Source: three-view drawing plus pictorial views. Frame: mm from the lowest corner of the part. A direction names the side the tool comes from. Coordinates: 2 decimals unless noted, no trailing zeros. Order: outer loops, then holes, each group sorted by start corner. A loop starts at its lowest first (then second) coordinate and runs counter-clockwise, first axis right, second up. Notation, with made-up numbers: M 61,-6 L 91,-6 A24 ccw 91,23 Z; hole C 2.25,54.25 d4. An arc over 180 degrees is marked long. Use CSV: the item, a comma, the result in double quotes. Start each with the question number.
Q1. Section query C-C, the plane x = 10.5. Output: boundary loops of the cut face in (y, z).
Q2. First-contact query: P1, Ø16, axis at x = 26, z = 25, coming from the +Y side; P2, Ø3, axis at x = 18, z = 24.5, coming from the -Y side. Flat tips, straight axial feed; report the tip coordinate or a pass-through.
Q3. Ray query, probe 1 along Y at (x, z) = (30, 7.5); probe 2 along X at (y, z) = (25, 12); probe 3 along Y at (x, z) = (34, 25.5). Return the intervals inside material, ascending.
Q4. Section query B-B, the plane z = 25. Output: boundary loops of the cut face in (x, y).
Q5. Section query D-D, the plane y = 16.5. Output: boundary loops of the cut face in (x, z), and give its area (3 significant figures).
Q6. Access query for the marked faces 1, 2 and 3. Directions: +Z, -Z, +X, -X, +Y, -Y. A direction counts if a zero-diameter tool reaches every point of the face in a straight line with its end or side. Return the directions, or none.
Q7. Section query A-A, the plane x = 26. Output: boundary loops of the cut face in (y, z).
Q8. Mould query, pull axis Y, two halves, no side actions, for the marked faces 4, 5 and 6. Classes: +Y half, -Y half, draft (parallel to the pull), parting line (faces both ways), or undercut.
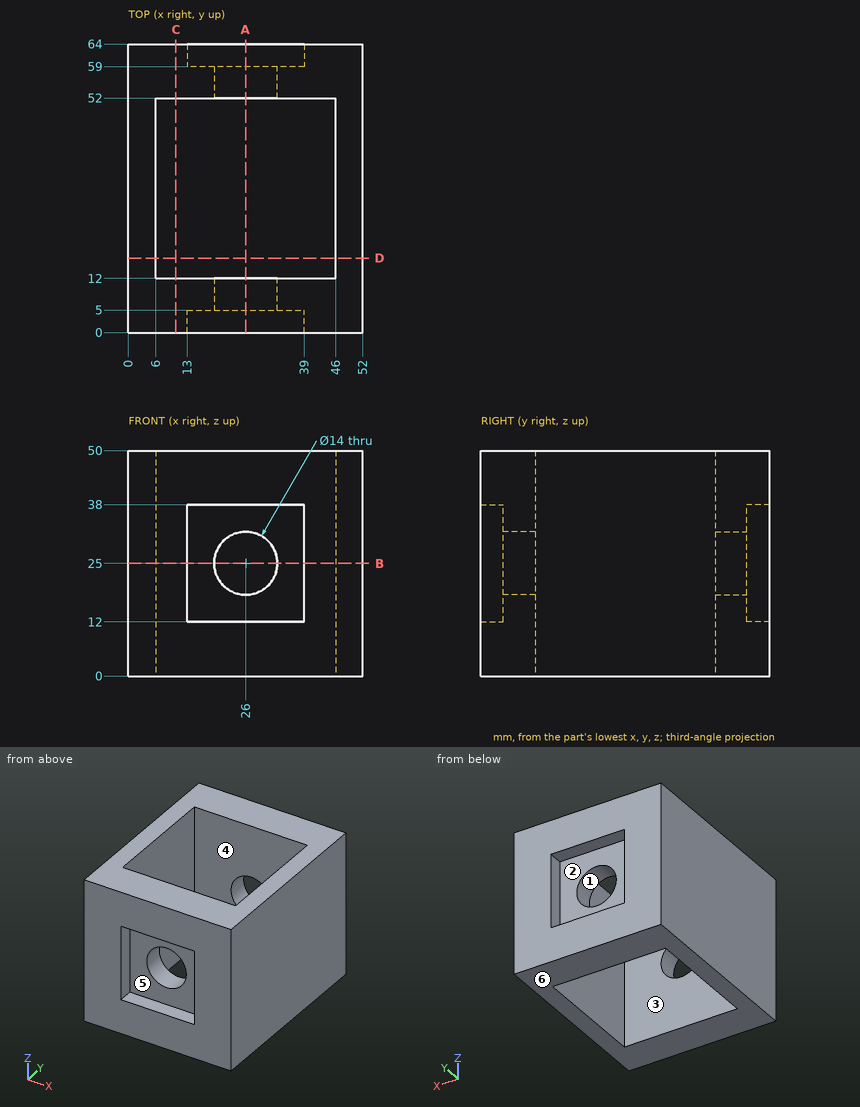
Responses:
1,outline,"M 0,0 L 12,0 L 12,50 L 0,50 Z; M 52,0 L 64,0 L 64,50 L 52,50 Z"
2,P1,"stops at y = 59"
2,P2,"stops at y = 5"
3,probe 1,"y = 0 to 12, 52 to 64"
3,probe 2,"x = 0 to 6, 46 to 52"
3,probe 3,"y = 5 to 12, 52 to 59"
4,outline,"M 0,0 L 13,0 L 13,5 L 19,5 L 19,12 L 6,12 L 6,52 L 19,52 L 19,59 L 13,59 L 13,64 L 0,64 Z; M 33,5 L 39,5 L 39,0 L 52,0 L 52,64 L 39,64 L 39,59 L 33,59 L 33,52 L 46,52 L 46,12 L 33,12 Z"
5,outline,"M 0,0 L 6,0 L 6,50 L 0,50 Z; M 46,0 L 52,0 L 52,50 L 46,50 Z"
5,area,"600 mm²"
6,face 1,"+Y, -Y"
6,face 2,"+Y"
6,face 3,"+Z, -Z"
7,outline,"M 0,0 L 12,0 L 12,18 L 5,18 L 5,12 L 0,12 Z; M 0,38 L 5,38 L 5,32 L 12,32 L 12,50 L 0,50 Z; M 52,0 L 64,0 L 64,12 L 59,12 L 59,18 L 52,18 Z; M 52,32 L 59,32 L 59,38 L 64,38 L 64,50 L 52,50 Z"
8,face 4,"undercut"
8,face 5,"-Y half"
8,face 6,"draft"
